Here's how the part is built. I have some questions about the finished solid (model axes, mm). A direction names the side the tool comes from. Round coordinates to 2 decimals unless told otherwise and drop trailing zeros. Write each loop counter-clockwise with the first axis right and the second up, starting at its lowest first coordinate (ties: lowest second). Pieces come first, ordered by that corner, then holes. Notation, with made-up numbers: (43, 7) - (83, 7) arc R30 ccw to (83, 30) - close; hole circle Ø5 at (50, -1). An arc over 180 degrees is marked (long way). One line per question, with ' | ' between items. Start each with the question number.
(1) Thinking about a two-plate mould opening in X: for faces 4 (the cylindrical face through (132.57, -4.2, 35.39)), 5 (the flat face through (139.12, -16, 39)), 6 (the flat face through (46.951, -61, 85)), 7 (the flat face through (-2, 54.143, 50)), which applies, pulls with the +X half, pulls with the -X half, needs draft (parallel to the pull), parting line crosses it, or undercut?
(2) For faces 1 (the flat face through (-46.951, -61, 85)), 2 (the flat face through (-2, -67.127, 50)), 3 (the flat face through (-125.841, -13, 39)), which set-ups out of +Z, -Z, +X, -X, +Y, -Y let a thin tool reach every point of the face, with its end or its side?
(3) Imagine slicing it at C-C (y = -49.5). Write out the boundary of the cut face in (x, z), plus the area to 3 significant figures.
(4) If I drill on L1, parallel to Y at x = 4, z = 4.5; L2, parallel to X at y = -42.5, z = 48; L3, parallel to X at y = -57.5, z = 86, over which ranges is the centre line in solid material (lowest first)?
(5) Imagine slicing it at B-B (x = -99.5). Write out the boundary of the cut face in (y, z).
(6) Imagine slicing it at D-D (z = 51). Write out the boundary of the cut face in (x, y), plus the area to 3 significant figures.
(7) Will this pin go through, and if not, where does the flat tip stop? pin 1 (10.5 mm diameter, centred on x = -18, y = 61.5, fed in from +Z).
(8) Imagine slicing it at A-A (y = 0). Write out the boundary of the cut face in (x, z), plus the area to 3 significant figures.
from build123d import *

# Parameters (mm, degrees)
F0_W     = 278.240532
F0_H     = 134.254978
F0_W_2   = 251.682728
F0_H_2   = 108.286024
F1_DEPTH = 101.6
F2_R     = 19.357944
F3_DEPTH = 278.241532
F4_W     = 93.901328
F4_H     = 31.952637
F5_DEPTH = 134.255977


with BuildPart() as f1:
    # F0 (on Top) → F1 (new body)
    with BuildSketch(Plane.XY):
        Rectangle(F0_W, F0_H)
        Rectangle(F0_W_2, F0_H_2, mode=Mode.SUBTRACT)
    extrude(amount=F1_DEPTH)

    # F2 (on face) → F3 (cut, through all)
    with BuildSketch(Plane.YZ.offset(139.120266)):
        with Locations((0, 54.288089)):
            Circle(F2_R)
    extrude(amount=-F3_DEPTH, mode=Mode.SUBTRACT)

    # F4 (on face) → F5 (cut, through all)
    with BuildSketch(Plane.XZ.offset(67.127489)):
        with Locations((0, 85.623682)):
            Rectangle(F4_W, F4_H)
    extrude(amount=-F5_DEPTH, mode=Mode.SUBTRACT)


solid = f1.part
Check sheet entries:
1) face 4: needs draft | face 5: pulls with the +X half | face 6: undercut | face 7: undercut
2) face 1: +Z, +Y, -Y | face 2: +Z, -Z, +X, -X, -Y | face 3: +Z, -Z
3) outline: (-139.12, 0) - (-125.84, 0) - (-125.84, 101.6) - (-139.12, 101.6) - close; (125.84, 0) - (139.12, 0) - (139.12, 101.6) - (125.84, 101.6) - close | area: 2,700 mm^2
4) L1: -67.13 to -54.14, 54.14 to 67.13 | L2: -139.12 to -125.84, 125.84 to 139.12 | L3: -139.12 to -46.95, 46.95 to 139.12
5) outline: (-67.13, 0) - (-54.14, 0) - (-54.14, 101.6) - (-67.13, 101.6) - close; (54.14, 0) - (67.13, 0) - (67.13, 101.6) - (54.14, 101.6) - close
6) outline: (-139.12, -67.13) - (139.12, -67.13) - (139.12, -19.08) - (125.84, -19.08) - (125.84, -54.14) - (-125.84, -54.14) - (-125.84, -19.08) - (-139.12, -19.08) - close; (-139.12, 19.08) - (-125.84, 19.08) - (-125.84, 54.14) - (125.84, 54.14) - (125.84, 19.08) - (139.12, 19.08) - (139.12, 67.13) - (-139.12, 67.13) - close | area: 9,090 mm^2
7) pin 1: z = 69.65
8) outline: (-139.12, 0) - (-125.84, 0) - (-125.84, 34.93) - (-139.12, 34.93) - close; (-139.12, 73.65) - (-125.84, 73.65) - (-125.84, 101.6) - (-139.12, 101.6) - close; (125.84, 0) - (139.12, 0) - (139.12, 34.93) - (125.84, 34.93) - close; (125.84, 73.65) - (139.12, 73.65) - (139.12, 101.6) - (125.84, 101.6) - close | area: 1,670 mm^2
